from build123d import *

# Parameters (mm, degrees)
F_3_3_3_3_DIAMETER_HOLE1_D     = 3.3
F_3_3_3_3_DIAMETER_HOLE1_DEPTH = 7.3
F_3_3_3_3_DIAMETER_HOLE1_TIP   = 0.991420021
CHAMFER1_SIZE                  = 0.55
CHAMFER2_SIZE                  = 0.3
FILLET1_R                      = 0.5
FILLET2_R                      = 1


with BuildPart() as part:
    # Sketch1 → Revolve1 (revolve)
    with BuildSketch(Plane.XY):
        with BuildLine():
            Line((-23.1, 3.307179677), (-23.1, 0))
            Line((-23.1, 0), (38.2, 0))
            Line((38.2, 0), (38.2, 3.653589838))
            Line((38.2, 3.653589838), (37.6, 4))
            Line((37.6, 4), (38, 4))
            Line((38, 4), (38, 30))
            Line((38, 30), (11.5, 30))
            Line((11.5, 30), (11.5, 29))
            Line((11.5, 29), (7.8, 29))
            Line((7.8, 29), (7.8, 32.000951614))
            Line((7.8, 32.000951614), (13.5, 32.2))
            Line((13.5, 32.2), (13.5, 33.2))
            Line((13.5, 33.2), (10.5, 33.2))
            Line((10.5, 33.2), (10.5, 33.98))
            Line((10.5, 33.98), (5, 33.98))
            Line((5, 33.98), (5, 34))
            Line((5, 34), (0, 34))
            Line((0, 34), (0, 11.288675135))
            Line((0, 11.288675135), (0.5, 11))
            Line((0.5, 11), (-2.6, 11))
            Line((-2.6, 11), (-2.6, 4.5))
            ThreePointArc((-2.6, 4.5), (-2.453553391, 4.146446609), (-2.1, 4))
            Line((-2.1, 4), (-21.9, 4))
            Line((-21.9, 4), (-23.1, 3.307179677))
        make_face()
    revolve(axis=Axis((-23.1, 0, 0), (1, 0, 0)))

    # Ø3.3 (3.3) Diameter Hole1
    with Locations(Plane.ZY):
        with Locations((0, 21.5), (18.619546181, -10.75), (-18.619546181, -10.75)):
            Hole(F_3_3_3_3_DIAMETER_HOLE1_D / 2, depth=F_3_3_3_3_DIAMETER_HOLE1_DEPTH)
            with Locations((0, 0, -(F_3_3_3_3_DIAMETER_HOLE1_DEPTH + F_3_3_3_3_DIAMETER_HOLE1_TIP / 2))):  # 118° drill point
                Cone(0, F_3_3_3_3_DIAMETER_HOLE1_D / 2, F_3_3_3_3_DIAMETER_HOLE1_TIP, mode=Mode.SUBTRACT)

    # Chamfer1
    chamfer1_edges = [part.edges().sort_by_distance(p)[0] for p in [
        (0, -10.75, -16.969546181),
        (0, -10.75, 20.269546181),
        (0, 21.5, 1.65),
    ]]
    chamfer(chamfer1_edges, length=CHAMFER1_SIZE)

    # Chamfer2
    chamfer2_edges = [part.edges().sort_by_distance(p)[0] for p in [
        (0, -34, 0),
    ]]
    chamfer(chamfer2_edges, length=CHAMFER2_SIZE)

    # Fillet1
    fillet1_edges = [part.edges().sort_by_distance(p)[0] for p in [
        (-2.6, -11, 0),
    ]]
    fillet(fillet1_edges, radius=FILLET1_R)

    # Fillet2
    fillet2_edges = [part.edges().sort_by_distance(p)[0] for p in [
        (-21.9, -4, 0),
        (38, -30, 0),
    ]]
    fillet(fillet2_edges, radius=FILLET2_R)


solid = part.part
Part model, mm, in its own coordinate system. A direction names the side the tool comes from. Give positions to 0.01 mm unless a question says otherwise; leave off trailing zeros. Use one line per item in the form item = value.
(1) Drill centre lines: line 1 (Z direction, x = 2, y = -10); line 2 (Y direction, x = 11, z = -23.5); line 3 (Y direction, x = 8, z = 22.5). Where is each one in solid material? Low to high. Write a range as from..to.
Solution:
line_1 = -32.5..-20.09, -17.15..17.15, 20.09..32.5
line_2 = -23.45..-21.89, -16.99..16.99, 21.89..23.45
line_3 = -25.46..-22.77, -18.3..18.3, 22.77..25.46
(2) Pull direction Y, two halves, no side cores. Call faces 4 (the face through (11.98, -7.2, -32.41)), 5 (the face through (3.972, 23.136, 0.215)), 6 (the face through (10.5, -33, -7)): +Y half, -Y half, draft (parallel to the pull), parting line (faces both ways), or undercut.
Solution:
face_4 = parting line
face_5 = undercut
face_6 = draft
(3) Flat gauge pins, fed straight in: P1, Ø4, axis at y = -19, z = 2.5, coming from the -X side; P2, Ø5.5, axis at y = -10.75, z = 18.62, coming from the +X side; P3, Ø6, axis at y = 1, z = 8.5, coming from the -X side. Where does each tip first touch, or does it go through?
Solution:
P1 = 0
P2 = 38
P3 = -2.6
(4) Tool access for faces 1 (the face through (11.5, -16, 25)), 2 (the face through (2.62, 18.28, 28.67)), 3 (the face through (3.97, -11.75, 19.93)): list every direction of +Z, -Z, +X, -X, +Y, -Y with a clear straight run to the whole face (end or side of a thin tool).
Solution:
face_1 = none
face_2 = +X, -X
face_3 = -X
